Autodesk Inventor part; units mm, degrees
ref_plane "YZ Plane" through (0, 0, 0) normal (1, 0, 0) x (0, 1, 0)
ref_plane "XZ Plane" through (0, 0, 0) normal (0, 1, 0) x (-1, 0, 0)
ref_plane "XY Plane" through (0, 0, 0) normal (0, 0, 1) x (1, 0, 0)
sketch "Sketch1" plane through (0, 0, 0) normal (1, 0, 0) x (0, 1, 0)
  line L0 (203.2, 185.3184) -> (203.2, 134.5184)
  line L1 (203.2, 134.5184) -> (0, -25.4)
  line L2 (0, -25.4) -> (0, 25.4)
  line L3 (0, 25.4) -> (203.2, 185.3184)
  line L4 (0, 0) -> (32.2745, 0) construction
  line L5 (203.2, 159.9184) -> (170.9255, 159.9184) construction
  line L6 (0, 25.4) -> (64.5489, 25.4) construction
  line L7 (203.2, 134.5184) -> (138.6511, 134.5184) construction
  circle A0 centre (196.85, 166.2684) radius 1.5875
  line L8 (203.2, 147.2184) -> (154.7883, 147.2184) construction
  line L9 (203.2, 166.2684) -> (178.9942, 166.2684) construction
  line L10 (196.85, 166.2684) -> (196.85, 147.2184) construction
  circle A1 centre (196.85, 147.2184) radius 1.5875
  circle A2 centre (177.8, 147.2184) radius 1.5875
  line L11 (0, -6.35) -> (24.2058, -6.35) construction
  line L12 (48.4117, 12.7) -> (0, 12.7) construction
  line L13 (6.35, -6.35) -> (6.35, 12.7) construction
  circle A3 centre (6.35, -6.35) radius 1.5875
  circle A4 centre (6.35, 12.7) radius 1.5875
  circle A5 centre (25.4, 12.7) radius 1.5875
  point P0 (0, 0)
  dimension "d0" = 50.8
  dimension "d4" = 159.9184
  dimension "d5" = 3.175
  dimension "d6" = 19.05
  dimension "d7" = 6.35
  dimension "d8" = 19.05
  dimension "d9" = 6.35
  dimension "d10" = 19.05
  dimension "d11" = 6.35
  dimension "d12" = 6.35
  dimension "d13" = 19.05
  dimension "d16" = 190.5
extrude "Extrusion1" add sketch "Sketch1" along normal blind 3.175
properties part number "Cross Brace"
CAD build for the part. Positions are in the model's coordinates, mm. Round coordinates to 2 decimals unless told otherwise and drop trailing zeros. Order: outer loops, then holes, each group sorted by start corner. A loop starts at its lowest first (then second) coordinate and runs counter-clockwise, first axis right, second up. Notation, with made-up numbers: (29, 63) - (39, 63) arc R21 ccw to (39, 98) - close; hole circle Ø7 at (47, 53). An arc over 180 degrees is marked (long way). Return JSON: item names as keys, results as strings.
(1) Cut at A-A (y = 190). Give the cut face in (x, z) (3 decimals), then the cut area to 3 significant figures.
Answer key:
{"outline": "(0, 124.13) - (3.175, 124.13) - (3.175, 174.93) - (0, 174.93) - close", "area": "161 mm^2"}
(2) Pin check, flat tips, straight feed: pin 1 Ø2.5 at (y, z) = (196.85, 147.22) entering from +X; pin 2 Ø1 at (x, z) = (2, 92.5) entering from +Y. Stop position of each tip, or through.
Answer key:
{"pin 1": "passes through", "pin 2": "stops at y = 150.44"}
(3) Cut at B-B (z = 57). Give the cut face in (x, y) (3 decimals).
Answer key:
{"outline": "(0, 40.152) - (3.175, 40.152) - (3.175, 104.701) - (0, 104.701) - close"}
(4) Wall check: probe 1 along Z at (x, y) = (0.75, 196.85); probe 2 along Y at (x, z) = (2.8, -6); probe 3 along Z at (x, y) = (2.1, 177.8). Give the ranges that are in metal, low to high. Write a range as from..to.
Answer key:
{"probe 1": "z = 129.52..145.63, 148.81..164.68, 167.86..180.32", "probe 2": "y = 0..4.8, 7.9..24.65", "probe 3": "z = 114.53..145.63, 148.81..165.33"}
